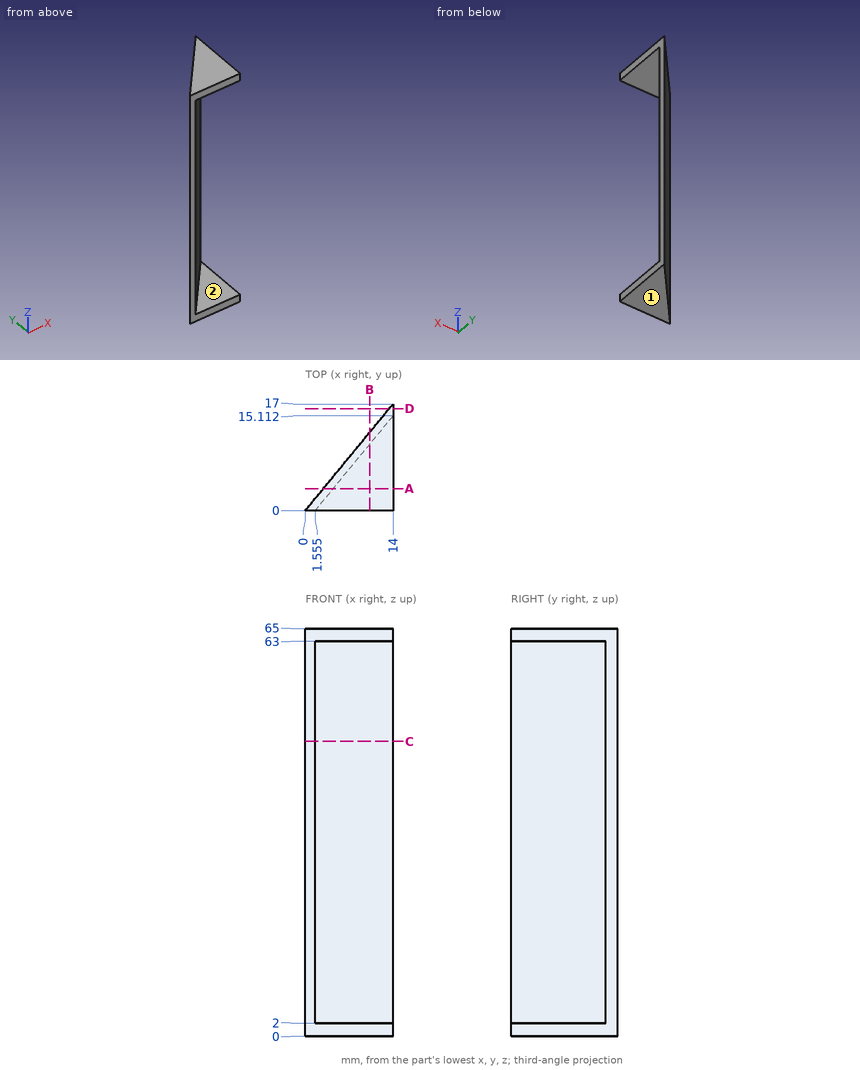
Could you check a few things on this drawing? It's one solid part, dimensions in mm from its lowest x, y, z. A direction names the side the tool comes from. Coordinates: 2 decimals unless noted, no trailing zeros. Order: outer loops, then holes, each group sorted by start corner. A loop starts at its lowest first (then second) coordinate and runs counter-clockwise, first axis right, second up. Notation, with made-up numbers: (22.5, 64.5) - (31.5, 64.5) arc R15 ccw to (31.5, 87.5) - close; hole circle Ø6 at (53.5, -23.5). An arc over 180 degrees is marked (long way). Answer as a JSON object with one key per item and string values. Group by question number.
Q1. Imagine slicing it at D-D (y = 16.25). Please give me the cut outline in (x, z).
Q2. Imagine slicing it at C-C (z = 47). Please give me the cut outline in (x, y) (1 decimal).
Q3. Imagine slicing it at A-A (y = 3.5). Please give me the cut outline in (x, z), and give its area (3 significant figures).
Q4. I need wall thicknesses on line 1 (Z direction, x = 3.75, y = 2); line 2 (X direction, y = 6.5, z = 32) (1 decimal); line 3 (X direction, y = 3.5, z = 16) (1 decimal). Which ranges of each line are inside material? Lowest first, please. Write a range as from..to.
Q5. Imagine slicing it at B-B (x = 10.25). Please give me the cut outline in (y, z), and give its area (3 significant figures).
Q6. Will these pins go through, and if not, where does the flat tip stop? P1, Ø6, axis at x = 12.5, z = 41.5, coming from the -Y side; P2, Ø4, axis at y = 13.5, z = 27.5, coming from the -X side; P3, Ø1.5, axis at x = 8.5, y = 13.5, coming from the -Z side; P4, Ø1.5, axis at x = 10, z = 14.5, coming from the +Y side (1 decimal).
Q7. On a 3-axis mill with a long thin cutter (end or side, diameter ignored), from which of +Z, -Z, +X, -X, +Y, -Y can I reach the whole of each face in a straight line? I mean the marked faces 1 and 2. Say none if no direction works.
Determined:
{
 "1": {"outline": "(13.38, 0) - (14, 0) - (14, 65) - (13.38, 65) - close"},
 "2": {"outline": "(0, 0) - (1.6, 0) - (14, 15.1) - (14, 17) - close"},
 "3": {"outline": "(2.88, 0) - (14, 0) - (14, 2) - (4.44, 2) - (4.44, 63) - (14, 63) - (14, 65) - (2.88, 65) - close", "area": "139 mm2"},
 "4": {"line 1": "z = 0..2, 63..65", "line 2": "x = 5.4..6.9", "line 3": "x = 2.9..4.4"},
 "5": {"outline": "(0, 0) - (12.45, 0) - (12.45, 65) - (0, 65) - (0, 63) - (10.56, 63) - (10.56, 2) - (0, 2) - close", "area": "165 mm2"},
 "6": {"P1": "stops at y = 9.65", "P2": "stops at x = 9.47", "P3": "passes through", "P4": "stops at y = 13.1"},
 "7": {"face 1": "-Z, +X, -X, +Y, -Y", "face 2": "+X, -Y"}
}
